Input: part model. Units: mm. Frame: model coordinates. Coordinates: 2 decimals unless noted, no trailing zeros. Order: outer loops, then holes, each group sorted by start corner. A loop starts at its lowest first (then second) coordinate and runs counter-clockwise, first axis right, second up. Notation, with made-up numbers: (42.25, 32) -> (48.25, 32) arc R29 ccw to (48.25, 56) -> close; hole circle Ø6 at (-4, -17.5). An arc over 180 degrees is marked (long way). Write each question's results on one line, items separated by ' | '.
```python
from build123d import *

# Parameters (mm, degrees)
SKETCH1_W           = 60
SKETCH1_H           = 75
BOSS_EXTRUDE1_DEPTH = 3.175
SKETCH2_R           = 1.45
CUT_EXTRUDE1_DEPTH  = 4.175
SKETCH3_R           = 6.3
SKETCH3_R_2         = 1.425
CUT_EXTRUDE2_DEPTH  = 4.175


with BuildPart() as part:
    # Sketch1 → Boss-Extrude1 (new body)
    with BuildSketch(Plane(origin=(0, 0, 0), x_dir=(1, 0, 0), z_dir=(0, 1, 0))):
        Rectangle(SKETCH1_W, SKETCH1_H)
    extrude(amount=BOSS_EXTRUDE1_DEPTH)

    # Sketch2 → Cut-Extrude1 (cut, through all)
    with BuildSketch(Plane(origin=(0, 3.175, 0), x_dir=(1, 0, 0), z_dir=(0, 1, 0))):
        with Locations((25, 32.5)):
            Circle(SKETCH2_R)
        with Locations((-25, 32.5)):
            Circle(SKETCH2_R)
        with Locations((15, 32.5)):
            Circle(SKETCH2_R)
        with Locations((25, -32.5)):
            Circle(SKETCH2_R)
        with Locations((15, -32.5)):
            Circle(SKETCH2_R)
        with Locations((-25, -32.5)):
            Circle(SKETCH2_R)
    extrude(amount=-CUT_EXTRUDE1_DEPTH, mode=Mode.SUBTRACT)

    # Sketch3 → Cut-Extrude2 (cut, through all)
    with BuildSketch(Plane(origin=(0, 3.175, 0), x_dir=(-1, 0, 0), z_dir=(0, 1, 0))):
        with Locations((12, -15)):
            Circle(SKETCH3_R)
        with Locations((12, 15)):
            Circle(SKETCH3_R)
        with Locations((-15, 20)):
            Circle(SKETCH3_R_2)
        with Locations((-15, 15)):
            Circle(SKETCH3_R_2)
        with Locations((-15, 10)):
            Circle(SKETCH3_R_2)
    extrude(amount=-CUT_EXTRUDE2_DEPTH, mode=Mode.SUBTRACT)


solid = part.part
```
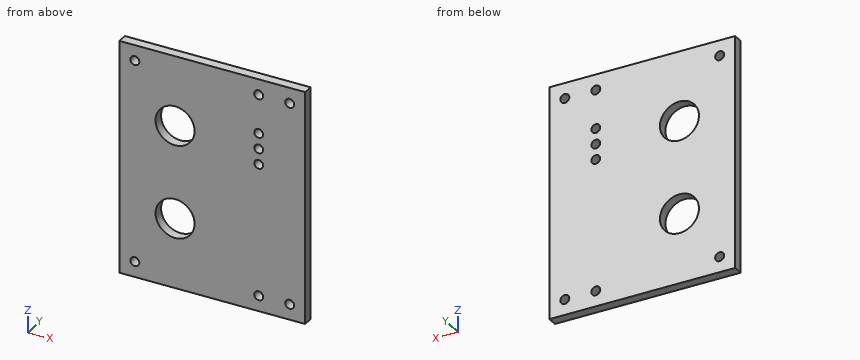
(1) Cut plane D-D, the plane x = 25. Return loops of the section in (y, z) (3 decimals), plus the area to 3 significant figures.
Return value:
outline: (0, -37.5) -> (3.175, -37.5) -> (3.175, -33.95) -> (0, -33.95) -> close; (0, -31.05) -> (3.175, -31.05) -> (3.175, 31.05) -> (0, 31.05) -> close; (0, 33.95) -> (3.175, 33.95) -> (3.175, 37.5) -> (0, 37.5) -> close | area: 220 mm2
(2) Cut plane A-A, the plane x = -12. Return loops of the section in (y, z) (3 decimals), plus the area to 3 significant figures.
Return value:
outline: (0, -37.5) -> (3.175, -37.5) -> (3.175, -21.3) -> (0, -21.3) -> close; (0, -8.7) -> (3.175, -8.7) -> (3.175, 8.7) -> (0, 8.7) -> close; (0, 21.3) -> (3.175, 21.3) -> (3.175, 37.5) -> (0, 37.5) -> close | area: 158 mm2
(3) Pin query (flat end, axial travel): P1, Ø2.5, axis at x = 15, z = 15, coming from the -Y side. Return the tip coordinate at first contact, or that it passes through.
Return value:
P1: through
(4) Cut plane B-B, the plane y = 0.95. Count the separate pieces of the cut face and the enclosed holes in it, plus the area to 3 significant figures.
Return value:
separate pieces: 1 | enclosed holes: 11 | area: 4,190 mm2
(5) Cut plane C-C, the plane z = -12. Return loops of the section in (x, y) (3 decimals), plus the area to 3 significant figures.
Return value:
outline: (-30, 0) -> (-17.54, 0) -> (-17.54, 3.175) -> (-30, 3.175) -> close; (-6.46, 0) -> (30, 0) -> (30, 3.175) -> (-6.46, 3.175) -> close | area: 155 mm2
(6) Line query: line 1 along Z through (x, y) = (15, 1.5) (3 decimals); line 2 along X through (y, z) = (0.75, 32.5); line 3 along Z through (x, y) = (-12, 0.7). Output: solid intervals per line, ascending. Write a range as from..to.
Return value:
line 1: -37.5..-33.95, -31.05..8.575, 11.425..13.575, 16.425..18.575, 21.425..31.05, 33.95..37.5 | line 2: -30..-26.45, -23.55..13.55, 16.45..23.55, 26.45..30 | line 3: -37.5..-21.3, -8.7..8.7, 21.3..37.5
